from build123d import *

# Parameters (mm, degrees)
F1_DEPTH = 58.5
F3_DEPTH = 148.4
F4_R     = 2
F5_DEPTH = 25
F6_W     = 5
F6_H     = 20
F7_DEPTH = 50.5
F8_SIZE  = 3


with BuildPart() as f1:
    # F0 (on Right) → F1 (new body, symmetric)
    with BuildSketch(Plane.YZ):
        Polygon((36.5, -7.5), (36.5, 17.5), (-36.5, 17.5), (-36.5, -7.5), (-51.5, -7.5), (-51.5, -17.5), (-36.5, -17.5), (-21.5, -17.5), (-21.5, 2.5), (21.5, 2.5), (21.5, -17.5), (36.5, -17.5), (51.5, -17.5), (51.5, -7.5), align=None)
    extrude(amount=F1_DEPTH, both=True)

    # F2 (on Front) → F3 (cut)
    with BuildSketch(Plane.XZ):
        with BuildLine():
            Line((-15, -17.5), (15, -17.5))
            ThreePointArc((15, -17.5), (0, -2.5), (-15, -17.5))
        make_face()
    extrude(amount=-F3_DEPTH, mode=Mode.SUBTRACT)

    # F4 (on Top) → F5 (cut)
    with BuildSketch(Plane.XY):
        with Locations((-34.84017, -44)):
            Circle(F4_R)
        with Locations((34.84017, -44)):
            Circle(F4_R)
        with Locations((-34.84017, 44)):
            Circle(F4_R)
        with Locations((34.84017, 44)):
            Circle(F4_R)
    extrude(amount=-F5_DEPTH, mode=Mode.SUBTRACT)

    # F6 (on Right) → F7 (cut, symmetric)
    with BuildSketch(Plane.YZ):
        with Locations((24, -7.5)):
            Rectangle(F6_W, F6_H)
        with Locations((-24, -7.5)):
            Rectangle(F6_W, F6_H)
    extrude(amount=F7_DEPTH, both=True, mode=Mode.SUBTRACT)

    # F8
    f8_edges = [f1.edges().sort_by_distance(p)[0] for p in [
        (0, 36.5, 17.5),
        (-58.5, 0, 17.5),
        (58.5, 0, 17.5),
        (0, -36.5, 17.5),
    ]]
    chamfer(f8_edges, length=F8_SIZE)


solid = f1.part
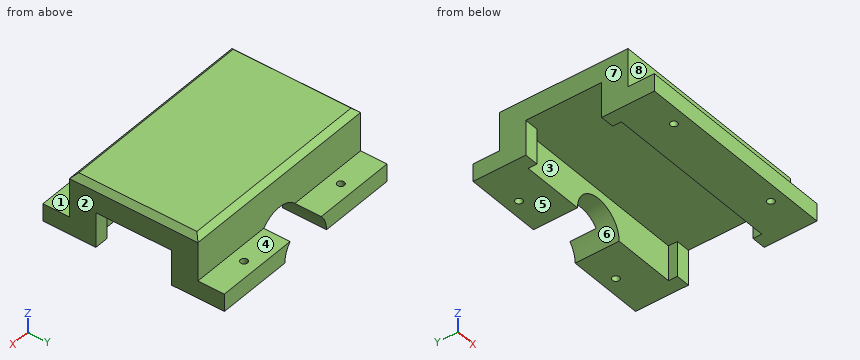
Work out the finished part from the listing and answer in its coordinate system (mm). Face numbers are marked on the shaded views. A direction names the side the tool comes from. Round coordinates to 2 decimals unless told otherwise and drop trailing zeros. Write each loop counter-clockwise with the first axis right and the second up, starting at its lowest first coordinate (ties: lowest second). Pieces come first, ordered by that corner, then holes. Notation, with made-up numbers: (-8.75, -12) - (35.25, -12) arc R29 ccw to (35.25, 19) - close; hole circle Ø5 at (-6.5, -14.75). An arc over 180 degrees is marked (long way). Answer in a Markdown table with one row per item. Add a question column.
1. A cutting plane is placed at B-B, the plane y = -44. Determine the outline of the cut face in (x, z).
2. A cutting plane is placed at C-C, the plane x = -16.5. Determine the outline of the cut face in (y, z).
3. For the marked faces 1, 2, 3, 4 and 5, determine the directions among +Z, -Z, +X, -X, +Y, -Y from which every point of the face is accessible in a straight line to the end or side of a thin tool.
4. Given pin 1 (16 mm diameter, centred on x = -12, y = -1, fed in from -Z); pin 2 (6.5 mm diameter, centred on x = -20, z = 1.5, fed in from +Y); pin 3 (2.5 mm diameter, centred on x = -34.84, y = 44, fed in from -Z); pin 4 (4 mm diameter, centred on x = 55, z = -3.5, fed in from -Y), each flat-ended and moving along its own axis, determine where each tip first touches the part or whether it passes through.
5. A cutting plane is placed at D-D, the plane y = 44. Determine the outline of the cut face in (x, z).
6. Find the intervals of material crossed by line 1 along Y through (x, z) = (21, 1.5); line 2 along Y through (x, z) = (21.5, -10); line 3 along Y through (x, z) = (40, 6), in increasing order. Write a range as from..to.
7. A cutting plane is placed at A-A, the plane z = 0.5. Determine the outline of the cut face in (x, y).
8. The mould has two halves that part along X. Classify the marked faces 6, 7 and 8: +X half, -X half, draft (parallel to the pull), parting line (faces both ways), or undercut.
Worked out:
| question | item | result |
|---|---|---|
| 1 | outline | (-58.5, -17.5) - (-36.84, -17.5) - (-36.84, -7.5) - (-58.5, -7.5) - close; (-32.84, -17.5) - (32.84, -17.5) - (32.84, -7.5) - (-32.84, -7.5) - close; (36.84, -17.5) - (58.5, -17.5) - (58.5, -7.5) - (36.84, -7.5) - close |
| 2 | outline | (-51.5, -17.5) - (-26.5, -17.5) - (-26.5, 2.5) - (26.5, 2.5) - (26.5, -17.5) - (51.5, -17.5) - (51.5, -7.5) - (36.5, -7.5) - (36.5, 14.5) - (33.5, 17.5) - (-33.5, 17.5) - (-36.5, 14.5) - (-36.5, -7.5) - (-51.5, -7.5) - close |
| 3 | face 1 | +Z, +X, -X, -Y |
| 3 | face 2 | +Z, -Z, +X, +Y, -Y |
| 3 | face 3 | -Z |
| 3 | face 4 | +Z, +X, -X, +Y |
| 3 | face 5 | -Z, +X, -X, +Y, -Y |
| 4 | pin 1 | z = 2.5 |
| 4 | pin 2 | y = 36.5 |
| 4 | pin 3 | through |
| 4 | pin 4 | y = -36.5 |
| 5 | outline | (-58.5, -17.5) - (-36.84, -17.5) - (-36.84, -7.5) - (-58.5, -7.5) - close; (-32.84, -17.5) - (-15, -17.5) arc R15 cw to (-11.18, -7.5) - (-32.84, -7.5) - close; (11.18, -7.5) arc R15 cw to (15, -17.5) - (32.84, -17.5) - (32.84, -7.5) - close; (36.84, -17.5) - (58.5, -17.5) - (58.5, -7.5) - (36.84, -7.5) - close |
| 6 | line 1 | -36.5..-26.5, 26.5..36.5 |
| 6 | line 2 | -51.5..-26.5, 26.5..51.5 |
| 6 | line 3 | -36.5..36.5 |
| 7 | outline | (-58.5, -36.5) - (58.5, -36.5) - (58.5, -21.5) - (50.5, -21.5) - (50.5, -26.5) - (-50.5, -26.5) - (-50.5, -21.5) - (-58.5, -21.5) - close; (-58.5, 21.5) - (-50.5, 21.5) - (-50.5, 26.5) - (50.5, 26.5) - (50.5, 21.5) - (58.5, 21.5) - (58.5, 36.5) - (-58.5, 36.5) - close |
| 8 | face 6 | undercut |
| 8 | face 7 | -X half |
| 8 | face 8 | draft |
